Input: part model. Units: mm. Frame: model coordinates. A direction names the side the tool comes from. Round coordinates to 2 decimals unless told otherwise and drop trailing zeros. Order: outer loops, then holes, each group sorted by start corner. A loop starts at its lowest first (then second) coordinate and runs counter-clockwise, first axis right, second up.
Item 1: Cut plane B-B on x = 1.5. Output: boundary loops of the cut face in (y, z) (3 decimals), then the cut area to 3 significant figures.
Item 2: Cut plane C-C on z = 8.5. Output: boundary loops of the cut face in (x, y) (3 decimals).
Item 3: First-contact query: pin 1 (1 mm diameter, centred on x = -12, z = 25, fed in from -Y); pin 2 (11.5 mm diameter, centred on x = 6.5, y = -1.5, fed in from -Z) (3 decimals); pin 3 (2 mm diameter, centred on x = -16, y = 23, fed in from -Z). Flat tips, straight axial feed; report the tip coordinate or a pass-through.
Item 4: Reachability of faces 1 (the flat face through (0, 79.375, 15)), 2 (the flat face through (-19.177, 1, 2)), 3 (the flat face through (-17.78, -1, 15)) from +Z, -Z, +X, -X, +Y, -Y: full face, straight path, thin tool, end or side. Return the list, or none.
Item 5: Cut plane A-A on y = 7.5. Output: boundary loops of the cut face in (x, z) (3 decimals).
Item 6: Line query: L1, parallel to X at y = 27, z = 18 (3 decimals); L2, parallel to X at y = 73.5, z = 2.5 (3 decimals); L3, parallel to Z at x = -8.5, y = -46 (3 decimals). Output: solid intervals per line, ascending.
Item 7: Mould query, pull axis X, two halves, no side actions, for faces 4 (the flat face through (1, -79.375, 30)), 5 (the flat face through (17.78, -4, 15)), 6 (the cylindrical face through (-19.529, -3.576, 31.516)). Classes: released by +X, released by -X, zero draft, split by the parting line, or undercut.
```python
from build123d import *

# Parameters (mm, degrees)
F1_DEPTH = 33.02
F2_R     = 5
F3_T     = -3.175
F4_W     = 38.354
F4_H     = 201.6773819923
F5_DEPTH = 3.175


with BuildPart() as f1:
    # F0 (on Top) → F1 (new body)
    with BuildSketch(Plane.XY):
        with BuildLine():
            ThreePointArc((20.955, 74.375), (19.4905339059, 77.9105339059), (15.955, 79.375))
            Line((15.955, 79.375), (-15.955, 79.375))
            ThreePointArc((-15.955, 79.375), (-19.4905339059, 77.9105339059), (-20.955, 74.375))
            Line((-20.955, 74.375), (-20.955, -79.375))
            Line((-20.955, -79.375), (20.955, -79.375))
            Line((20.955, -79.375), (20.955, 74.375))
        make_face()
    extrude(amount=F1_DEPTH)

    # F2
    f2_edges = [f1.edges().sort_by_distance(p)[0] for p in [
        (-20.955, -2.5, 33.02),
        (0, 79.375, 33.02),
    ]]
    fillet(f2_edges, radius=F2_R)

    # F3
    f3_openings = [f1.faces().sort_by_distance(p)[0] for p in [
        (0, -79.375, 16.389713),
        (0, -0.126416, 0),
    ]]
    offset(amount=F3_T, openings=f3_openings)

    # F4 (on face) → F5 (cut)
    with BuildSketch(Plane(origin=(0, 0, 0), x_dir=(1, 0, 0), z_dir=(0, 0, -1))):
        Rectangle(F4_W, F4_H)
    extrude(amount=-F5_DEPTH, mode=Mode.SUBTRACT)


solid = f1.part
```
From the geometry:
1. outline: (-79.375, 29.845) - (74.375, 29.845) arc R1.825 cw to (76.2, 28.02) - (76.2, 3.175) - (79.375, 3.175) - (79.375, 28.02) arc R5 ccw to (74.375, 33.02) - (-79.375, 33.02) - close
1. area: 584 mm2
2. outline: (-20.955, -79.375) - (-17.78, -79.375) - (-17.78, 74.375) arc R1.825 cw to (-15.955, 76.2) - (15.955, 76.2) arc R1.825 cw to (17.78, 74.375) - (17.78, -79.375) - (20.955, -79.375) - (20.955, 74.375) arc R5 ccw to (15.955, 79.375) - (-15.955, 79.375) arc R5 ccw to (-20.955, 74.375) - close
3. pin 1: stops at y = 76.2
3. pin 2: stops at z = 29.845
3. pin 3: stops at z = 29.52
4. face 1: +Z, -Z, +X, -X, +Y
4. face 2: -Z, +Y, -Y
4. face 3: -Z, -Y
5. outline: (-20.955, 0) - (-19.177, 0) - (-19.177, 3.175) - (-17.78, 3.175) - (-17.78, 28.02) arc R1.825 cw to (-15.955, 29.845) - (15.955, 29.845) arc R1.825 cw to (17.78, 28.02) - (17.78, 3.175) - (19.177, 3.175) - (19.177, 0) - (20.955, 0) - (20.955, 28.02) arc R5 ccw to (15.955, 33.02) - (-15.955, 33.02) arc R5 ccw to (-20.955, 28.02) - close
6. L1: x = -20.955 to -17.78, 17.78 to 20.955
6. L2: x = -20.955 to -19.177, 19.177 to 20.955
6. L3: z = 29.845 to 33.02
7. face 4: zero draft
7. face 5: undercut
7. face 6: released by -X
